from build123d import *

# Parameters (mm, degrees)
F0_W      = 97.79
F0_H      = 45.72
F1_DEPTH  = 101.6
F2_W      = 91.44
F2_H      = 95.25
F3_DEPTH  = 43.18
F4_W      = 19.05
F4_H      = 6.35
F5_ANGLE  = 180
F7_DEPTH  = 25.4
F8_R      = 3.17499
F10_D     = 6.35
F10_DEPTH = 101.601


# Not quite as in the source:
# - a fillet or chamfer is up to 0.001 mm smaller than in the source, because OpenCascade refuses the exact size


with BuildPart() as f1:
    # F0 (on Front) → F1 (new body)
    with BuildSketch(Plane.XZ):
        with Locations((15.4838143581, 4.6649015626)):
            Rectangle(F0_W, F0_H)
    extrude(amount=-F1_DEPTH)

    # F2 (on face) → F3 (cut)
    with BuildSketch(Plane.XY.offset(27.5249015626)):
        with Locations((15.4838143581, 50.8)):
            Rectangle(F2_W, F2_H)
    extrude(amount=-F3_DEPTH, mode=Mode.SUBTRACT)

    # F4 (on face) → F5 (revolve)
    with BuildSketch(Plane.XZ):
        with Locations((5.9588143581, 6.8874015626)):
            Rectangle(F4_W, F4_H)
        with Locations((5.9588143581, 0.5374015626)):
            Rectangle(F4_W, F4_H)
    revolve(axis=Axis((15.4838143581, 0, 3.7124015626), (0, 0, 1)), revolution_arc=F5_ANGLE)

    # F6 (on face) → F7 (cut)
    with BuildSketch(Plane.XY.offset(10.0624015626)):
        with BuildLine():
            Line((28.1838143581, 0), (2.7838143581, 0))
            ThreePointArc((2.7838143581, 0), (15.4838143581, -12.7), (28.1838143581, 0))
        make_face()
    extrude(amount=-F7_DEPTH, mode=Mode.SUBTRACT)

    # F8 (radius 3.175 in the source; OpenCascade refuses exactly that, so slightly less here)
    f8_edges = [f1.edges().sort_by_distance(p)[0] for p in [
        (15.483814, -19.05, 10.062402),
        (15.483814, -12.7, 10.062402),
        (15.483814, -19.05, -2.637598),
        (15.483814, -12.7, -2.637598),
    ]]
    fillet(f8_edges, radius=F8_R)

    # F10 (through all, one way)
    with BuildSketch(Plane.XZ):
        with Locations((15.4838143581, 2.1249015626)):
            Circle(F10_D / 2)
    extrude(amount=-F10_DEPTH, mode=Mode.SUBTRACT)


solid = f1.part
Here's how the part is built. I have some questions about the finished solid (model axes, mm). A direction names the side the tool comes from. Round coordinates to 2 decimals unless told otherwise and drop trailing zeros. Order: outer loops, then holes, each group sorted by start corner. A loop starts at its lowest first (then second) coordinate and runs counter-clockwise, first axis right, second up. Notation, with made-up numbers: (28, -28.75) -> (68, -28.75) arc R20 ccw to (68, 8.25) -> close; hole circle Ø4 at (-15, 88). An arc over 180 degrees is marked (long way). Return JSON: item names as keys, results as strings.
Q1. I need wall thicknesses on line 1 along X through (y, z) = (83.5, 22); line 2 along Y through (x, z) = (41, -8) (3 decimals); line 3 along Z through (x, y) = (0, 32.5). Which ranges of each line are inside material? Lowest first, please. Write a range as from..to.
Filled sheet:
{"line 1": "x = -33.41..-30.24, 61.2..64.38", "line 2": "y = 0..3.175, 98.425..101.6", "line 3": "z = -18.2..-15.66"}
Q2. For pin 1 Ø8 at (x, y) = (21.5, -9) entering from -Z; pin 2 Ø7.5 at (x, z) = (15.48, 2.12) entering from -Y; pin 3 Ø8 at (x, z) = (50, 1) entering from -Y, each with a flat end and sliding along its axis, tell me the tip position at first contact or that it passes through.
Filled sheet:
{"pin 1": "stops at z = -2.46", "pin 2": "stops at y = -19.05", "pin 3": "stops at y = 0"}
Q3. If we section it at D-D on x = 14.5: Give the number of separate pieces and of enclosed holes in the cut face, plus the area to 3 significant figures.
Filled sheet:
{"separate pieces": "4", "enclosed holes": "0", "area": "566 mm^2"}
Q4. If we mould it in two halves opening along X, with no side actions, what happens to faces 1 (the flat face through (-32, 51, 27.525)), 2 (the flat face through (64.379, 50, 4)), 3 (the flat face through (15, 98.425, 6))? For each: released by +X, released by -X, zero draft, split by the parting line, or undercut.
Filled sheet:
{"face 1": "zero draft", "face 2": "released by +X", "face 3": "undercut"}
Q5. If we section it at C-C on y = 10: List the corners of the cut face in (x, z) for me, plus the area to 3 significant figures.
Filled sheet:
{"outline": "(-33.41, -18.2) -> (64.38, -18.2) -> (64.38, 27.52) -> (61.2, 27.52) -> (61.2, -15.66) -> (-30.24, -15.66) -> (-30.24, 27.52) -> (-33.41, 27.52) -> close", "area": "523 mm^2"}
Q6. If we section it at A-A on z = 13.5: List the corners of the cut face in (x, y) for me (3 decimals).
Filled sheet:
{"outline": "(-33.411, 0) -> (64.379, 0) -> (64.379, 101.6) -> (-33.411, 101.6) -> close; hole (-30.236, 3.175) -> (61.204, 3.175) -> (61.204, 98.425) -> (-30.236, 98.425) -> close"}
Q7. Which directions (+Z, -Z, +X, -X, +Y, -Y) give clear straight access to the entire face, cutting with the end or side of a thin tool? Please do faces 4 (the cylindrical face through (18.417, 99.99, 0.909)), 5 (the flat face through (15, 3.175, 6)), 6 (the cylindrical face through (15.205, -12.697, 3.757)), 7 (the cylindrical face through (15.065, -19.045, 3.668)).
Filled sheet:
{"face 4": "+Y", "face 5": "+Z", "face 6": "+Z, -Z", "face 7": "+Z, -Z, -Y"}
Q8. If we section it at B-B on x = -8: List the corners of the cut face in (y, z) for me (3 decimals).
Filled sheet:
{"outline": "(0, -18.195) -> (101.6, -18.195) -> (101.6, 27.525) -> (98.425, 27.525) -> (98.425, -15.655) -> (3.175, -15.655) -> (3.175, 27.525) -> (0, 27.525) -> close"}
